```python
from build123d import *

# Parameters (mm, degrees)
SKETCH_W     = 55
SKETCH_H     = 25
SKETCH_W_2   = 15
SKETCH_H_2   = 15
PAD_DEPTH    = 10
SKETCH001_W  = 15.5
SKETCH001_H  = 15.5
POCKET_DEPTH = 10.001


with BuildPart() as part:
    # Sketch → Pad (new body)
    with BuildSketch(Plane.XY):
        with Locations((22.5, 7.5)):
            Rectangle(SKETCH_W, SKETCH_H)
        with Locations((7.5, 7.5)):
            Rectangle(SKETCH_W_2, SKETCH_H_2, mode=Mode.SUBTRACT)
        with Locations((37.5, 7.5)):
            Rectangle(SKETCH_W_2, SKETCH_H_2, mode=Mode.SUBTRACT)
    extrude(amount=PAD_DEPTH)

    # Sketch001 (on Face14 of Pad) → Pocket (cut, through all)
    with BuildSketch(Plane.XY.offset(10)):
        with Locations((7.5, 7.5)):
            Rectangle(SKETCH001_W, SKETCH001_H)
        with Locations((37.5, 7.5)):
            Rectangle(SKETCH001_W, SKETCH001_H)
    extrude(amount=-POCKET_DEPTH, mode=Mode.SUBTRACT)


solid = part.part
```
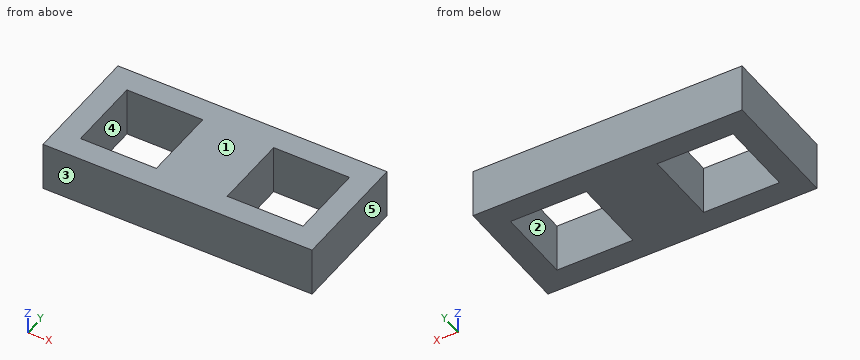
Geometry check sheet. Reference: the model listing, model coordinates, mm. Face numbers are marked on the shaded views. A direction names the side the tool comes from. Round coordinates to 2 decimals unless told otherwise and drop trailing zeros. Order: outer loops, then holes, each group sorted by start corner. A loop starts at its lowest first (then second) coordinate and runs counter-clockwise, first axis right, second up. Notation, with made-up numbers: (-4, -24.5) - (42, -24.5) arc R18 ccw to (42, -11.5) - close; hole circle Ø4 at (35.25, 5). An arc over 180 degrees is marked (long way). Use a Markdown table: item, result. Add a question column.
(1) Depth check by flat-ended pin: pin 1 (12 mm diameter, centred on x = 40, y = 3.5, fed in from -Z). Enter the tip coordinate at first touch or a pass-through.
(2) Tool access check on the marked faces 1 and 2. Record the directions out of +Z, -Z, +X, -X, +Y, -Y that give a thin tool (end or side, any length) a straight path to the whole face; none if there is none.
(3) Material ranges on line 1 along X through (y, z) = (14.25, 0.5); line 2 along Y through (x, z) = (9.5, 5.75), recorded low to high. Write a range as [from, to].
(4) Sectioned sample at C-C, the plane z = 6. Enter the section's corners in (x, y).
(5) Release check for a two-part mould opening along X. For the marked faces 3, 4 and 5 record: pulls with the +X half, pulls with the -X half, needs draft (parallel to the pull), parting line crosses it, or undercut.
(6) Sectioned sample at B-B, the plane x = 40.5. Enter the section's corners in (y, z).
(7) Sectioned sample at A-A, the plane y = 0.75. Enter the section's corners in (x, z), and give its area (3 significant figures).
Answers below:
| question | item | result |
|---|---|---|
| 1 | pin 1 | z = 0 |
| 2 | face 1 | +Z, +X, -X, +Y, -Y |
| 2 | face 2 | +Z, -Z |
| 3 | line 1 | [-5, -0.25], [15.25, 29.75], [45.25, 50] |
| 3 | line 2 | [-5, -0.25], [15.25, 20] |
| 4 | outline | (-5, -5) - (50, -5) - (50, 20) - (-5, 20) - close; hole (-0.25, -0.25) - (15.25, -0.25) - (15.25, 15.25) - (-0.25, 15.25) - close; hole (29.75, -0.25) - (45.25, -0.25) - (45.25, 15.25) - (29.75, 15.25) - close |
| 5 | face 3 | needs draft |
| 5 | face 4 | undercut |
| 5 | face 5 | pulls with the +X half |
| 6 | outline | (-5, 0) - (-0.25, 0) - (-0.25, 10) - (-5, 10) - close; (15.25, 0) - (20, 0) - (20, 10) - (15.25, 10) - close |
| 7 | outline | (-5, 0) - (-0.25, 0) - (-0.25, 10) - (-5, 10) - close; (15.25, 0) - (29.75, 0) - (29.75, 10) - (15.25, 10) - close; (45.25, 0) - (50, 0) - (50, 10) - (45.25, 10) - close |
| 7 | area | 240 mm² |
